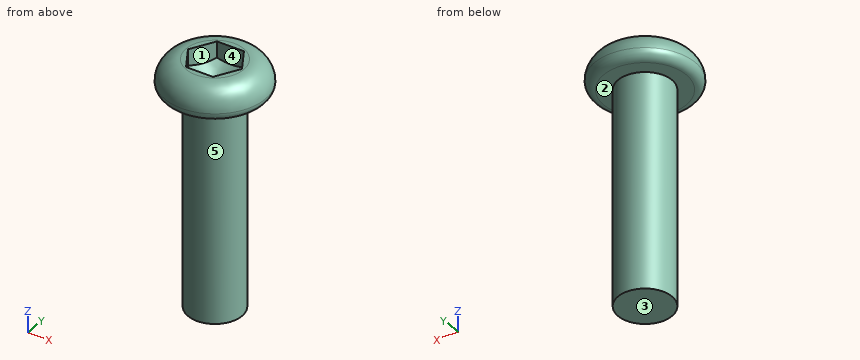
Autodesk Inventor part; units mm, degrees
ref_plane "YZ Plane" through (0, 0, 0) normal (1, 0, 0) x (0, 1, 0)
ref_plane "XZ Plane" through (0, 0, 0) normal (0, 1, 0) x (-1, 0, 0)
ref_plane "XY Plane" through (0, 0, 0) normal (0, 0, 1) x (1, 0, 0)
sketch "Sketch1" plane through (0, 0, 0) normal (0, 0, 1) x (1, 0, 0)
  circle A0 centre (0, 0) radius 2.8
  dimension "d0" = 5.6
extrude "Extrusion1" add sketch "Sketch1" along normal blind 1.7
fillet "Fillet3" radius 0.5 1 edges at (-2.8, 0, 0)
fillet "Fillet4" radius 1.2 1 edges at (-2.8, 0, 1.7)
sketch "Sketch2" plane through (0, 0, 1.7) normal (0, 0, 1) x (1, 0, 0)
  line L0 (-0.75, -1.299) -> (0.75, -1.299)
  line L1 (0.75, -1.299) -> (1.5, 0)
  line L2 (1.5, 0) -> (0.75, 1.299)
  line L3 (0.75, 1.299) -> (-0.75, 1.299)
  line L4 (-0.75, 1.299) -> (-1.5, 0)
  line L5 (-1.5, 0) -> (-0.75, -1.299)
  dimension "d7" = 3
extrude "Extrusion2" cut sketch "Sketch2" against normal blind 1.7
sketch "Sketch3" plane through (0, 0, 0) normal (0, 1, 0) x (-1, 0, 0)
  line L0 (0, 0) -> (1.5, 0)
  line L1 (2.3, 0) -> (-2.3, 0)
  line L2 (1.5, 0) -> (1.5, 0.8)
  line L3 (1.5, 0.8) -> (0, 0)
  line L4 (0, 0) -> (0, 2.432)
  dimension "d13" = 0
  dimension "d14" = 1.5
  dimension "d15" = 0.8
revolve "Revolution2" add sketch "Sketch3" angle 360 about axis through (0, 0, 0) along (0, 0, 1)
sketch "Sketch4" plane through (0, 0, 0) normal (0, 0, -1) x (-1, 0, 0)
  circle A0 centre (0, 0) radius 2.3
  circle A1 centre (0, 0) radius 1.5
  dimension "d18" = 3
extrude "Extrusion3" add sketch "Sketch4" along normal blind 12 contours A1
thread "Thread1"
properties part number "screw_M3_12_hex"
Design review of the part built by this model. Coordinates are the model's own, in mm. Face numbers are marked on the shaded views. A direction names the side the tool comes from. Coordinates: 2 decimals unless noted, no trailing zeros. Order: outer loops, then holes, each group sorted by start corner. A loop starts at its lowest first (then second) coordinate and runs counter-clockwise, first axis right, second up. Notation, with made-up numbers: (13, -35.75) -> (72, -35.75) arc R20 cw to (72, -5.75) -> close; hole circle Ø5 at (-18.75, -12.75). An arc over 180 degrees is marked (long way). One line per item, written item: value. Start each with the question number.
Q1. Tool access review of the marked faces 1 and 2: name each direction out of +Z, -Z, +X, -X, +Y, -Y from which nothing blocks a thin tool from reaching the whole face with its end or side.
Q2. For probe 1 along X at (y, z) = (0.15, 1.25); probe 2 along Z at (x, y) = (1.5, 0.65); probe 3 along Y at (x, z) = (0.25, -6), list the stretches that pass through material, from the lowest coordinate up.
Q3. Take a section at A-A, the plane z = -10.5. State the section outline as (x, y) points.
Q4. Mouldability with a two-part tool opening along Y and no side actions: class the marked faces 3, 4 and 5 as pulls with the +Y half, pulls with the -Y half, needs draft (parallel to the pull), parting line crosses it, or undercut.
Q5. Insertion check: pin 1 Ø1.5 at (y, z) = (-1.5, -2.5) entering from -X; pin 2 Ø3 at (x, z) = (1, -4) entering from +Y; pin 3 Ø2 at (y, z) = (-0.5, -4) entering from -X. Each pin has a flat end and moves straight along its axis. Give the tip position at first contact, or say it passes through.
Values follow:
1. face 1: +Z
1. face 2: -Z
2. probe 1: x = -2.53 to -1.41, 1.41 to 2.53
2. probe 2: z = 0 to 1.7
2. probe 3: y = -1.48 to 1.48
3. outline: circle Ø3 at (0, 0)
4. face 3: needs draft
4. face 4: undercut
4. face 5: parting line crosses it
5. pin 1: stops at x = -1.3
5. pin 2: stops at y = 1.5
5. pin 3: stops at x = -1.5
